The listing builds one solid part. Answer for the finished solid, in the listing's coordinates (mm). Face numbers are marked on the shaded views. A direction names the side the tool comes from. Give positions to 0.01 mm unless a question says otherwise; leave off trailing zeros. Order: outer loops, then holes, each group sorted by start corner. A loop starts at its lowest first (then second) coordinate and runs counter-clockwise, first axis right, second up. Notation, with made-up numbers: (45.5, -34) - (66.5, -34) arc R14 cw to (66.5, -20) - close; hole circle Ø6 at (-9.75, -19). An arc over 180 degrees is marked (long way). Answer as a JSON object with one key per item and string values. Group by question number.
Q1. For the marked faces 1, 2 and 3, determine the directions among +Z, -Z, +X, -X, +Y, -Y from which every point of the face is accessible in a straight line to the end or side of a thin tool.
Q2. Consider line 1 (Z direction, x = 26.5, y = 1.25); line 2 (Y direction, x = -34, z = -5); line 3 (Z direction, x = -35, y = 2). Determine where each line is inside the solid, lowest interval first.
Q3. A cutting plane is placed at A-A, the plane x = 11. Give the vertices of the cut face in (y, z), and give its area (3 significant figures).
Q4. Given pin 1 (3 mm diameter, centred on x = -32.5, y = 2.5, fed in from -Z); pin 2 (1.5 mm diameter, centred on y = 2.93, z = -5, fed in from -X), each flat-ended and moving along its own axis, determine where each tip first touches the part or whether it passes through.
Q5. A cutting plane is placed at B-B, the plane y = 5.25. Count the separate pieces of the cut face and the enclosed holes in it, and give its area (3 significant figures).
Q6. A cutting plane is placed at C-C, the plane x = -31. Give the vertices of the cut face in (y, z).
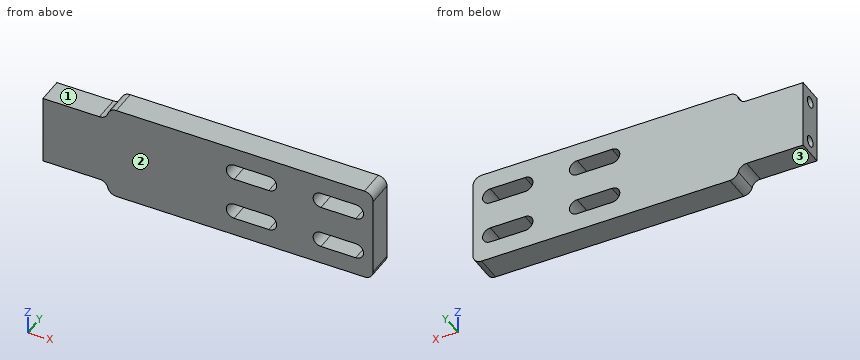
from build123d import *

# Parameters (mm, degrees)
BOSS_EXTRUDE1_DEPTH      = 6
M3_CLEARANCE_SLOT1_DEPTH = 6
M3_TAPPED_HOLE1_D        = 2.5
M3_TAPPED_HOLE1_DEPTH    = 8.5
M3_TAPPED_HOLE1_TIP      = 0.751075774
FILLET1_R                = 2


# Read off the part's stored shape, not the designer's step: M3 Clearance Slot1
with BuildPart() as part:
    # Sketch1 → Boss-Extrude1 (new body)
    with BuildSketch(Plane(origin=(0, 0, 0), x_dir=(1, 0, 0), z_dir=(0, 1, 0))):
        with BuildLine():
            Line((36, 11), (-23, 11))
            Line((-23, 11), (-23, 10))
            ThreePointArc((-23, 10), (-23.585786438, 8.585786438), (-25, 8))
            Line((-25, 8), (-38, 8))
            Line((-38, 8), (-38, -8))
            Line((-38, -8), (-25, -8))
            ThreePointArc((-25, -8), (-23.585786438, -8.585786438), (-23, -10))
            Line((-23, -10), (-23, -11))
            Line((-23, -11), (36, -11))
            ThreePointArc((36, -11), (37.414213562, -10.414213562), (38, -9))
            Line((38, -9), (38, 9))
            ThreePointArc((38, 9), (37.414213562, 10.414213562), (36, 11))
        make_face()
    extrude(amount=BOSS_EXTRUDE1_DEPTH)

    # M3 Clearance Slot1 outline → M3 Clearance Slot1 (cut)
    with BuildSketch(Plane(origin=(0, 0, 0), x_dir=(1, 0, 0), z_dir=(0, 1, 0))):
        with BuildLine():
            ThreePointArc((6, 6.8), (4.2, 5), (6, 3.2))
            Line((6, 3.2), (14, 3.2))
            ThreePointArc((14, 3.2), (15.8, 5), (14, 6.8))
            Line((14, 6.8), (6, 6.8))
        make_face()
        with BuildLine():
            ThreePointArc((34, 3.2), (35.8, 5), (34, 6.8))
            Line((34, 6.8), (26, 6.8))
            ThreePointArc((26, 6.8), (24.2, 5), (26, 3.2))
            Line((26, 3.2), (34, 3.2))
        make_face()
        with BuildLine():
            ThreePointArc((6, -3.2), (4.2, -5), (6, -6.8))
            Line((6, -6.8), (14, -6.8))
            ThreePointArc((14, -6.8), (15.8, -5), (14, -3.2))
            Line((14, -3.2), (6, -3.2))
        make_face()
        with BuildLine():
            ThreePointArc((34, -6.8), (35.8, -5), (34, -3.2))
            Line((34, -3.2), (26, -3.2))
            ThreePointArc((26, -3.2), (24.2, -5), (26, -6.8))
            Line((26, -6.8), (34, -6.8))
        make_face()
    extrude(amount=M3_CLEARANCE_SLOT1_DEPTH, mode=Mode.SUBTRACT)

    # M3 Tapped Hole1
    with Locations(Plane.ZY.offset(38)):
        with Locations((-5, 2.934782609), (5, 2.934782609)):
            Hole(M3_TAPPED_HOLE1_D / 2, depth=M3_TAPPED_HOLE1_DEPTH)
            with Locations((0, 0, -(M3_TAPPED_HOLE1_DEPTH + M3_TAPPED_HOLE1_TIP / 2))):  # 118° drill point
                Cone(0, M3_TAPPED_HOLE1_D / 2, M3_TAPPED_HOLE1_TIP, mode=Mode.SUBTRACT)

    # Fillet1
    fillet1_edges = [part.edges().sort_by_distance(p)[0] for p in [
        (-23, 3, 11),
        (-23, 3, -11),
    ]]
    fillet(fillet1_edges, radius=FILLET1_R)


solid = part.part
Reply:
{
 "1": {"face 1": "+Z, -X, +Y, -Y", "face 2": "+Z, -Z, +X, -X, -Y", "face 3": "-Z, -X, +Y, -Y"},
 "2": {"line 1": "z = -11 to -6.8, -3.2 to 3.2, 6.8 to 11", "line 2": "y = 0 to 1.68, 4.18 to 6", "line 3": "z = -8 to -5.83, -4.17 to 4.17, 5.83 to 8"},
 "3": {"outline": "(0, -11) - (6, -11) - (6, -6.8) - (0, -6.8) - close; (0, -3.2) - (6, -3.2) - (6, 3.2) - (0, 3.2) - close; (0, 6.8) - (6, 6.8) - (6, 11) - (0, 11) - close", "area": "88.8 mm^2"},
 "4": {"pin 1": "stops at z = -8", "pin 2": "stops at x = -29.2"},
 "5": {"separate pieces": "1", "enclosed holes": "4", "area": "1,420 mm^2"},
 "6": {"outline": "(0, -8) - (6, -8) - (6, 8) - (0, 8) - close; hole circle Ø2.5 at (2.93, -5); hole circle Ø2.5 at (2.93, 5)"}
}
